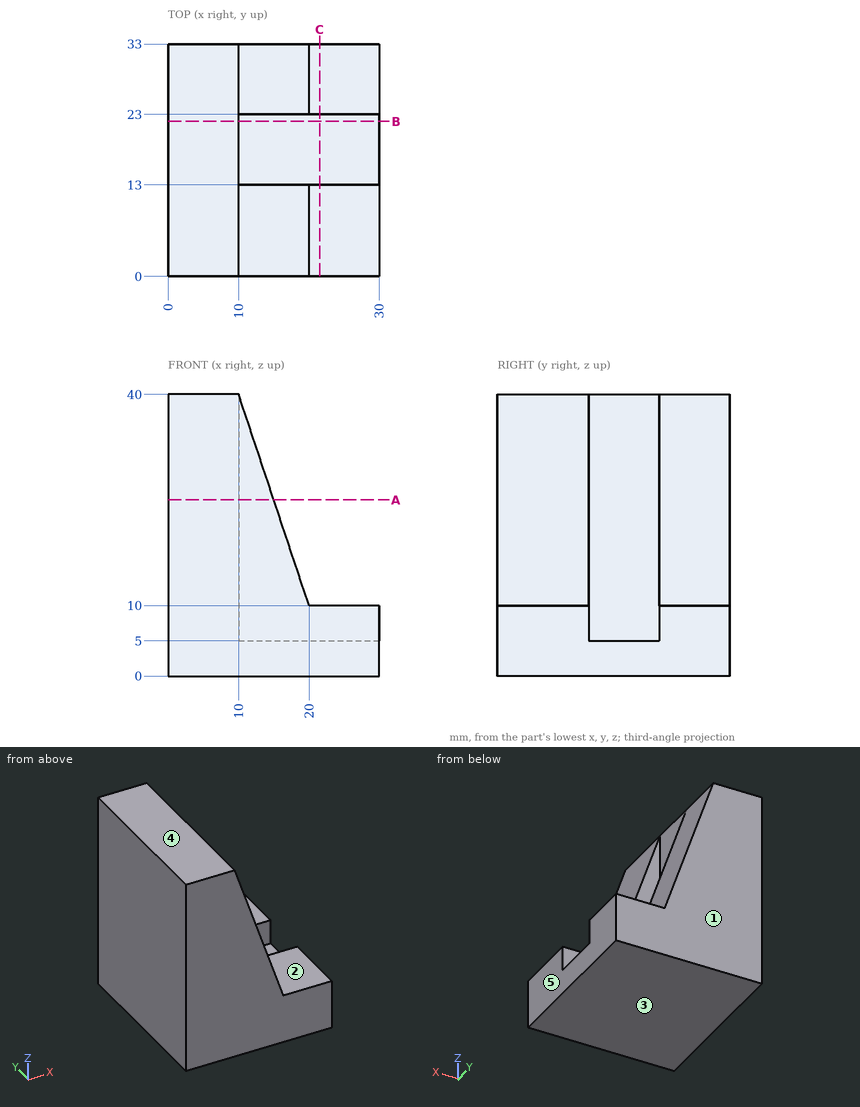
Can you work these out from the drawing? Everything is in mm from the part's minimum corner. A direction names the side the tool comes from. Round coordinates to 2 decimals unless told otherwise and drop trailing zeros. Write each loop counter-clockwise with the first axis right and the second up, starting at its lowest first coordinate (ties: lowest second). Pieces come first, ordered by that corner, then holes.
1. If we mould it in two halves opening along Z, with no side actions, what happens to the marked faces 3, 4 and 5? For each: released by +Z, released by -Z, zero draft, split by the parting line, or undercut.
2. Suppose I cut it at B-B (y = 22). List the corners of the cut face in (x, z) for me.
3. Suppose I cut it at C-C (x = 21.5). List the corners of the cut face in (y, z) for me.
4. Will these pins go through, and if not, where does the flat tip stop? pin 1 Ø3 at (x, y) = (25.5, 30) entering from +Z; pin 2 Ø8 at (y, z) = (15.5, 14.5) entering from +X.
5. Suppose I cut it at A-A (z = 25). List the corners of the cut face in (x, y) for me.
6. I need wall thicknesses on L1, parallel to Y at x = 13.5, z = 12.5; L2, parallel to Z at x = 26, y = 7. Which ranges of each line are inside material? Lowest first, please.
7. For the marked faces 1 and 2, which set-ups out of +Z, -Z, +X, -X, +Y, -Y let a thin tool reach every point of the face, with its end or its side?
Answer sheet:
1. face 3: released by -Z
1. face 4: released by +Z
1. face 5: zero draft
2. outline: (0, 0) - (30, 0) - (30, 5) - (10, 5) - (10, 40) - (0, 40) - close
3. outline: (0, 0) - (33, 0) - (33, 10) - (23, 10) - (23, 5) - (13, 5) - (13, 10) - (0, 10) - close
4. pin 1: stops at z = 10
4. pin 2: stops at x = 19.54
5. outline: (0, 0) - (15, 0) - (15, 13) - (10, 13) - (10, 23) - (15, 23) - (15, 33) - (0, 33) - close
6. L1: y = 0 to 13, 23 to 33
6. L2: z = 0 to 10
7. face 1: +Z, -Z, +X, -X, +Y
7. face 2: +Z, +X, +Y, -Y
